Could you check a few things on this model? Use its own coordinates, in mm. A direction names the side the tool comes from. Round coordinates to 2 decimals unless told otherwise and drop trailing zeros. Loops run counter-clockwise (first coordinate to the right, second up) from the corner with the lowest first, then second, coordinate; pieces in that order, holes last. Notation, with made-up numbers: (85, -38) -> (93, -38) arc R22 cw to (93, -10) -> close; hole circle Ø9 at (88, 35). An arc over 180 degrees is marked (long way). Write each question's results on one line, items separated by ' | '.
from build123d import *

# Parameters (mm, degrees)
CYLINDER007_R          = 2
CYLINDER007_DEPTH      = 5
CYLINDER007_ROLL_ANGLE = 15
CYLINDER004_R          = 2
CYLINDER004_DEPTH      = 5
CYLINDER004_ROLL_ANGLE = -15
CYLINDER006_R          = 2
CYLINDER006_DEPTH      = 5
CYLINDER006_ROLL_ANGLE = -15
BOX003_W               = 60
BOX003_H               = 28
BOX003_DEPTH           = 8
FILLET002_R            = 1
CYLINDER005_R          = 2
CYLINDER005_DEPTH      = 5
CYLINDER005_ROLL_ANGLE = 15


with BuildPart() as cylinder009:
    # Cylinder007 → Cylinder007 (new body)
    with BuildSketch(Plane.XY):
        Circle(CYLINDER007_R)
    extrude(amount=CYLINDER007_DEPTH)


with BuildPart() as cylinder009_1:
    # Cylinder007 roll: moved
    add(cylinder009.part.rotate(Axis((0, 0, 0), (1, 0, 0)), CYLINDER007_ROLL_ANGLE))


with BuildPart() as cylinder009_2:
    # Cylinder007 placement: moved
    add(cylinder009_1.part.moved(Location((48, 42.5, 5))))


with BuildPart() as cylinder:
    # Cylinder004 → Cylinder004 (new body)
    with BuildSketch(Plane.XY):
        Circle(CYLINDER004_R)
    extrude(amount=CYLINDER004_DEPTH)


with BuildPart() as cylinder_1:
    # Cylinder004 roll: moved
    add(cylinder.part.rotate(Axis((0, 0, 0), (1, 0, 0)), CYLINDER004_ROLL_ANGLE))


with BuildPart() as cylinder_2:
    # Cylinder004 placement: moved
    add(cylinder_1.part.moved(Location((48, 53.5, 5))))


with BuildPart() as cylinder008:
    # Cylinder006 → Cylinder006 (new body)
    with BuildSketch(Plane.XY):
        Circle(CYLINDER006_R)
    extrude(amount=CYLINDER006_DEPTH)


with BuildPart() as cylinder008_1:
    # Cylinder006 roll: moved
    add(cylinder008.part.rotate(Axis((0, 0, 0), (1, 0, 0)), CYLINDER006_ROLL_ANGLE))


with BuildPart() as cylinder008_2:
    # Cylinder006 placement: moved
    add(cylinder008_1.part.moved(Location((16, 53.5, 5))))


with BuildPart() as obj1:
    # Box003 → Box003 (new body)
    with BuildSketch(Plane.XY.offset(29)):
        with Locations((30, 14)):
            Rectangle(BOX003_W, BOX003_H)
    extrude(amount=BOX003_DEPTH)

    # Fillet002
    fillet002_edges = [obj1.edges().sort_by_distance(p)[0] for p in [
        (0, 0, 33),
        (0, 14, 37),
        (0, 28, 33),
        (0, 14, 29),
        (60, 0, 33),
        (60, 14, 37),
        (60, 28, 33),
        (60, 14, 29),
        (30, 0, 29),
        (30, 0, 37),
        (30, 28, 29),
        (30, 28, 37),
    ]]
    fillet(fillet002_edges, radius=FILLET002_R)


with BuildPart() as obj1_1:
    # Fillet002 placement: moved
    add(obj1.part.moved(Location((2, 34, -21))))


with BuildPart() as obj2:
    # Cylinder005 → Cylinder005 (new body)
    with BuildSketch(Plane.XY):
        Circle(CYLINDER005_R)
    extrude(amount=CYLINDER005_DEPTH)


with BuildPart() as obj2_1:
    # Cylinder005 roll: moved
    add(obj2.part.rotate(Axis((0, 0, 0), (1, 0, 0)), CYLINDER005_ROLL_ANGLE))


with BuildPart() as obj2_2:
    # Cylinder005 placement: moved
    add(obj2_1.part.moved(Location((16, 42.5, 5))))

    # Fusion003: union Cylinder009, Cylinder, Cylinder008, obj1
    add(cylinder009_2.part)
    add(cylinder_2.part)
    add(cylinder008_2.part)
    add(obj1_1.part)


solid = obj2_2.part
1) I'm going to push flat-ended pins straight in: pin 1 (8 mm diameter, centred on x = 36.5, y = 44.5, fed in from -Z); pin 2 (4 mm diameter, centred on y = 40.5, z = 6.5, fed in from -X). Where does each tip first touch, or does it pass through?
Model answer:
pin 1: stops at z = 8 | pin 2: stops at x = 2.13
2) If we mould it in two halves opening along X, with no side actions, what happens to faces 3 (the flat face through (32, 62, 12)), 4 (the cylindrical face through (15.57, 40.24, 5.88)), 5 (the cylindrical face through (47.74, 55.786, 5.87)), 6 (the flat face through (62, 48, 12))? For each: released by +X, released by -X, zero draft, split by the parting line, or undercut.
Model answer:
face 3: zero draft | face 4: undercut | face 5: undercut | face 6: released by +X
3) For faces 1 (the flat face through (16, 53.5, 5)), 2 (the flat face through (32, 48, 16)), which set-ups out of +Z, -Z, +X, -X, +Y, -Y let a thin tool reach every point of the face, with its end or its side?
Model answer:
face 1: -Z, +X, -X | face 2: +Z, +X, -X, +Y, -Y
4) I want a section at A-A, the plane y = 57.25. Write out the boundary of the cut face in (x, z).
Model answer:
outline: (2, 9) arc R1 ccw to (3, 8) -> (61, 8) arc R1 ccw to (62, 9) -> (62, 15) arc R1 ccw to (61, 16) -> (3, 16) arc R1 ccw to (2, 15) -> close
5) I want a section at B-B, the plane x = 20.5. Write out the boundary of the cut face in (y, z).
Model answer:
outline: (34, 9) arc R1 ccw to (35, 8) -> (61, 8) arc R1 ccw to (62, 9) -> (62, 15) arc R1 ccw to (61, 16) -> (35, 16) arc R1 ccw to (34, 15) -> close
6) I need wall thicknesses on line 1 (Z direction, x = 24.5, y = 38.25); line 2 (Y direction, x = 51, z = 8.5); line 3 (X direction, y = 57.5, z = 8.5). Which ranges of each line are inside material? Lowest first, please.
Model answer:
line 1: z = 8 to 16 | line 2: y = 34.13 to 61.87 | line 3: x = 2.13 to 61.87
